```python
from build123d import *
from OCP.BRepFilletAPI import BRepFilletAPI_MakeChamfer

# Parameters (mm, degrees)
T_LE_DE_BASE_PLI_E1_DEPTH = 0.3
CHANFREIN1_SIZE           = 0.4
CHANFREIN1_SIZE2          = 0.125


# Sheet-metal steps are written as plain solids
with BuildPart() as part:
    # Esquisse2 → Tôle de base pliée1 (new, symmetric)
    with BuildSketch(Plane(origin=(0, 0, 0), x_dir=(0, 0, -1), z_dir=(1, 0, 0))):
        with BuildLine():
            Line((-6, 0), (0, 0))
            Line((0, 0), (8.33, 0))
            ThreePointArc((8.33, 0), (8.931040764, -0.248959236), (9.18, -0.85))
            Line((9.18, -0.85), (9.18, -9.48))
            Line((9.18, -9.48), (8.58, -9.48))
            Line((8.58, -9.48), (8.58, -0.85))
            ThreePointArc((8.58, -0.85), (8.506776695, -0.673223305), (8.33, -0.6))
            Line((8.33, -0.6), (0, -0.6))
            Line((0, -0.6), (-6, -0.6))
            Line((-6, -0.6), (-6, 0))
        make_face()
    extrude(amount=T_LE_DE_BASE_PLI_E1_DEPTH, both=True)

    # Chanfrein1: one chamfer whose edges measure the first distance from different faces: ONE call of the kernel's chamfer builder (chamfer() names one face for all edges)
    chanfrein1_edges_1 = [part.edges().sort_by_distance(p)[0] for p in [
        (-0.3, -9.48, -8.88),
        (-0.3, -0.3, 6),
    ]]
    chanfrein1_side_1 = [part.faces().sort_by_distance(p)[0] for p in [
        (-0.3, -0.178970053, -1.165),
    ]]
    chanfrein1_edges_2 = [part.edges().sort_by_distance(p)[0] for p in [
        (0, -0.6, 6),
    ]]
    chanfrein1_side_2 = [part.faces().sort_by_distance(p)[0] for p in [
        (0, -0.6, -1.165),
    ]]
    chanfrein1_edges_3 = [part.edges().sort_by_distance(p)[0] for p in [
        (0, 0, 6),
    ]]
    chanfrein1_side_3 = [part.faces().sort_by_distance(p)[0] for p in [
        (0, 0, -1.165),
    ]]
    chanfrein1_edges_4 = [part.edges().sort_by_distance(p)[0] for p in [
        (0, -9.48, -9.18),
    ]]
    chanfrein1_side_4 = [part.faces().sort_by_distance(p)[0] for p in [
        (0, -5.165, -9.18),
    ]]
    chanfrein1_edges_5 = [part.edges().sort_by_distance(p)[0] for p in [
        (0, -9.48, -8.58),
    ]]
    chanfrein1_side_5 = [part.faces().sort_by_distance(p)[0] for p in [
        (0, -5.165, -8.58),
    ]]
    chanfrein1_edges_6 = [part.edges().sort_by_distance(p)[0] for p in [
        (0.3, -0.3, 6),
        (0.3, -9.48, -8.88),
    ]]
    chanfrein1_side_6 = [part.faces().sort_by_distance(p)[0] for p in [
        (0.3, -0.178970053, -1.165),
    ]]
    chanfrein1 = BRepFilletAPI_MakeChamfer(part.part.solid().wrapped)
    for e in chanfrein1_edges_1:
        chanfrein1.Add(CHANFREIN1_SIZE, CHANFREIN1_SIZE2, e.wrapped, chanfrein1_side_1[0].wrapped)  # the first distance lies on this face
    for e in chanfrein1_edges_2:
        chanfrein1.Add(CHANFREIN1_SIZE, CHANFREIN1_SIZE2, e.wrapped, chanfrein1_side_2[0].wrapped)  # the first distance lies on this face
    for e in chanfrein1_edges_3:
        chanfrein1.Add(CHANFREIN1_SIZE, CHANFREIN1_SIZE2, e.wrapped, chanfrein1_side_3[0].wrapped)  # the first distance lies on this face
    for e in chanfrein1_edges_4:
        chanfrein1.Add(CHANFREIN1_SIZE, CHANFREIN1_SIZE2, e.wrapped, chanfrein1_side_4[0].wrapped)  # the first distance lies on this face
    for e in chanfrein1_edges_5:
        chanfrein1.Add(CHANFREIN1_SIZE, CHANFREIN1_SIZE2, e.wrapped, chanfrein1_side_5[0].wrapped)  # the first distance lies on this face
    for e in chanfrein1_edges_6:
        chanfrein1.Add(CHANFREIN1_SIZE, CHANFREIN1_SIZE2, e.wrapped, chanfrein1_side_6[0].wrapped)  # the first distance lies on this face
    add(Compound.cast(chanfrein1.Shape()), mode=Mode.REPLACE)


solid = part.part
```
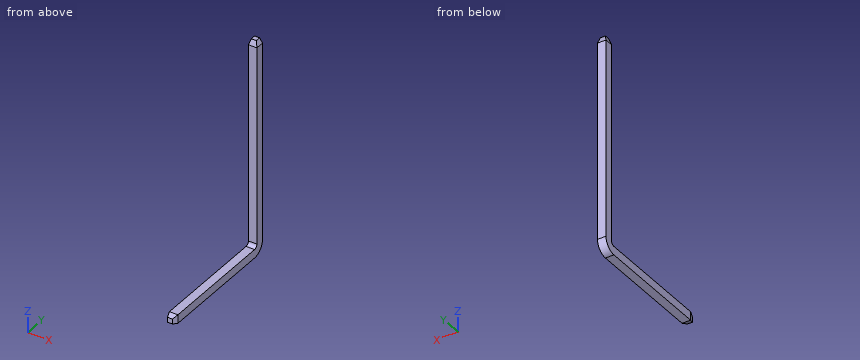
The listing builds one solid part. Answer for the finished solid, in the listing's coordinates (mm). Give positions to 0.01 mm unless a question says otherwise; leave off trailing zeros. Order: outer loops, then holes, each group sorted by start corner. A loop starts at its lowest first (then second) coordinate and runs counter-clockwise, first axis right, second up.
Item 1: The part is cut by section B-B, the plane z = 3. Give the vertices of the cut face in (x, y), and give its area (3 significant figures).
From the geometry:
outline: (-0.3, -0.6) - (0.3, -0.6) - (0.3, 0) - (-0.3, 0) - close
area: 0.360 mm2
Item 2: The part is cut by section C-C, the plane y = -6. Give the vertices of the cut face in (x, z).
From the geometry:
outline: (-0.3, -9.18) - (0.3, -9.18) - (0.3, -8.58) - (-0.3, -8.58) - close
Item 3: The part is cut by section A-A, the plane x = -0.05. Give the vertices of the cut face in (y, z) (3 decimals), and give its area (3 significant figures).
From the geometry:
outline: (-9.48, -9.055) - (-9.08, -9.18) - (-0.85, -9.18) arc R0.85 ccw to (0, -8.33) - (0, 5.6) - (-0.125, 6) - (-0.475, 6) - (-0.6, 5.6) - (-0.6, -8.33) arc R0.25 cw to (-0.85, -8.58) - (-9.08, -8.58) - (-9.48, -8.705) - close
area: 14.2 mm2
Item 4: Find the intervals of material crossed by probe 1 along Y at (x, z) = (-0.25, 5.25); probe 2 along Z at (x, y) = (0, -5.5), in increasing order.
From the geometry:
probe 1: y = -0.6 to 0
probe 2: z = -9.18 to -8.58
